Design review of the part built by this model. Coordinates are the model's own, in mm. Coordinates: 2 decimals unless noted, no trailing zeros. Order: outer loops, then holes, each group sorted by start corner. A loop starts at its lowest first (then second) coordinate and runs counter-clockwise, first axis right, second up. Notation, with made-up numbers: (35, 5) - (48, 5) arc R26 ccw to (48, 42) - close; hole circle Ø9 at (-27.5, 13.25). An arc over 180 degrees is marked (long way). Write item = value, one per line. Start each with the question number.
Autodesk Inventor part; units mm, degrees
ref_plane "YZ Plane" through (0, 0, 0) normal (1, 0, 0) x (0, 1, 0)
ref_plane "XZ Plane" through (0, 0, 0) normal (0, 1, 0) x (-1, 0, 0)
ref_plane "XY Plane" through (0, 0, 0) normal (0, 0, 1) x (1, 0, 0)
sketch "Sketch1" plane through (0, 0, 0) normal (0, 1, 0) x (-1, 0, 0)
  line L0 (0, 0) -> (-3, 0)
  line L1 (-3, 0) -> (-3, -70)
  line L2 (-3, -70) -> (0, -70)
  line L3 (0, -70) -> (0, 0)
  line L4 (0, -3) -> (0, 0)
  dimension "d0" = 3
  dimension "d1" = 70
extrude "Extrusion1" add sketch "Sketch1" along normal blind 60
sketch "Sketch2" plane through (3, 0, -3) normal (1, 0, 0) x (0, 0, -1)
  line L0 (67, 0) -> (-3, 0)
  line L1 (-3, 0) -> (37, 0) construction
  line L2 (37, 0) -> (37, 30) construction
  line L3 (37, 30) -> (-3, 30) construction
  line L4 (-3, 30) -> (-3, 0) construction
  circle A0 centre (37, 30) radius 25
  line L5 (37, 30) -> (62, 30) construction
  circle A1 centre (62, 30) radius 3.25
  circle A2 centre (24.5, 51.6506) radius 3.25
  circle A3 centre (24.5, 8.3494) radius 3.25
  circle A4 centre (37, 30) radius 12.5
  dimension "d8" = 50
  dimension "d6" = 30
  dimension "d7" = 40
  dimension "d9" = 6.5
  dimension "d12" = 360
  dimension "d36" = 25
hole "Hole1" at (3, 8.3494, -27.5) at (3, 51.6506, -27.5) at (3, 30, -65) direction (-1, 0, 0) diameter 6.5 depth 10
extrude "Extrusion2" cut sketch "Sketch2" against normal blind 50 contours A4
properties part number "motorbracket"
Item 1: Add section D-D on y = 38. Give the boundary of the cut face in (x, z), plus the area to 3 significant figures.
Item 2: For line 1 (Y direction, x = 1.15, z = -65); line 2 (Y direction, x = 1.3, z = -40); line 3 (Z direction, x = 0.4, y = 36), list the stretches that pass through material, from the lowest coordinate up.
Item 3: Mouldability with a two-part tool opening along Y and no side actions: class faces 1 (the flat face through (2, 0, -35)), 2 (the flat face through (3, 30, -27)), 3 (the cylindrical face through (1.479, 31.978, -62.421)) as +Y half, -Y half, draft (parallel to the pull), parting line (faces both ways), or undercut.
Item 4: Add section A-A on z = -65. Give the boundary of the cut face in (x, y).
Item 5: Add section B-B on y = 31. Give the boundary of the cut face in (x, z).
Item 6: For P1, Ø4, axis at y = 8.35, z = -27.5, coming from the -X side, flat-tipped, find the tip position at first contact; note if it passes through.
Item 7: Add section C-C on x = 0.85. Give the boundary of the cut face in (y, z).
Worked out:
q1.outline = (0, -70) - (3, -70) - (3, -49.6) - (0, -49.6) - close; (0, -30.4) - (3, -30.4) - (3, 0) - (0, 0) - close
q1.area = 152 mm2
q2.line_1 = 0 to 26.75, 33.25 to 60
q2.line_2 = 0 to 17.5, 42.5 to 60
q2.line_3 = -70 to -50.97, -29.03 to 0
q3.face_1 = -Y half
q3.face_2 = draft
q3.face_3 = undercut
q4.outline = (0, 0) - (3, 0) - (3, 26.75) - (0, 26.75) - close; (0, 33.25) - (3, 33.25) - (3, 60) - (0, 60) - close
q5.outline = (0, -70) - (3, -70) - (3, -68.09) - (0, -68.09) - close; (0, -61.91) - (3, -61.91) - (3, -52.46) - (0, -52.46) - close; (0, -27.54) - (3, -27.54) - (3, 0) - (0, 0) - close
q6.P1 = through
q7.outline = (0, -70) - (60, -70) - (60, 0) - (0, 0) - close; hole circle Ø6.5 at (8.35, -27.5); hole circle Ø25 at (30, -40); hole circle Ø6.5 at (30, -65); hole circle Ø6.5 at (51.65, -27.5)
